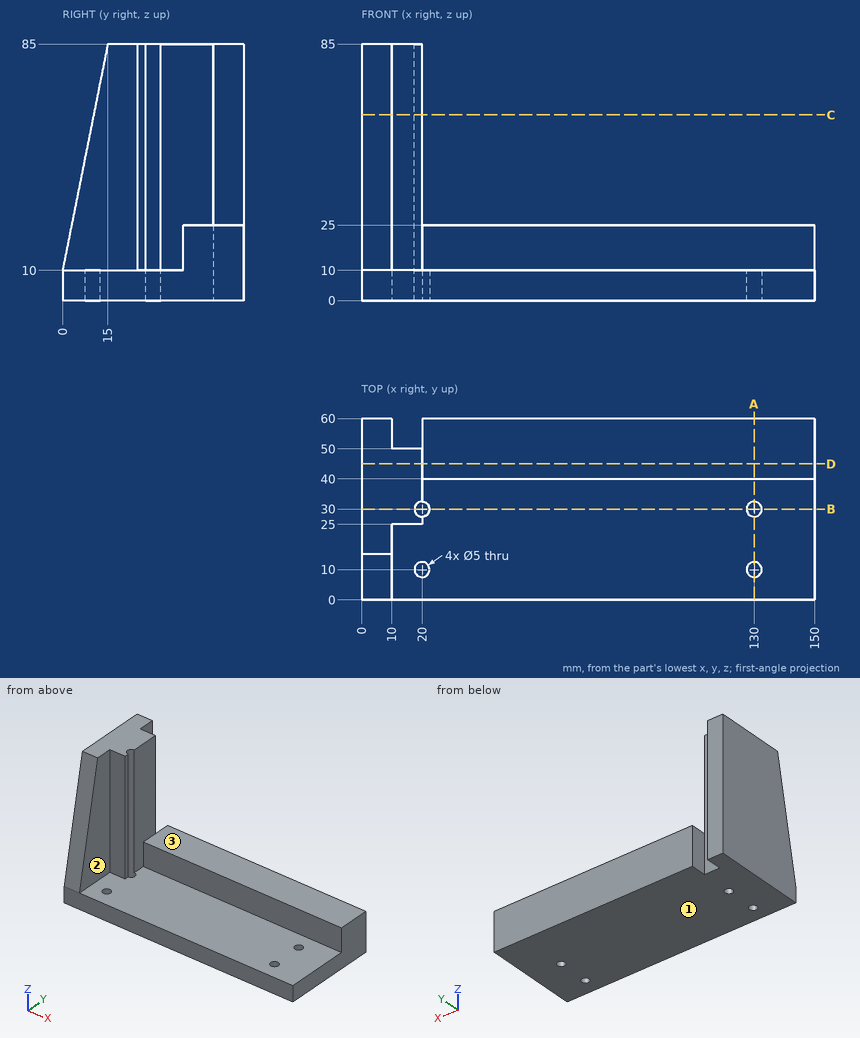
Study the drawing (mm; zero at the part's minimum x, y, z) and answer. A direction names the side the tool comes from. Coordinates: 2 decimals unless noted, no trailing zeros. Write each loop counter-clockwise with the first axis right and the second up, starting at its lowest first coordinate (ties: lowest second). Pieces come first, ordered by that corner, then holes. Notation, with made-up numbers: (-19, 5) - (5, 5) arc R29 cw to (5, 34) - close; hole circle Ø8 at (-30, 8). An arc over 180 degrees is marked (long way). One line per item, written item: value.
1) A tool of negligible diameter and unlimited length cuts with its end or side. For the marked faces 1, 2 and 3, from which of +Z, -Z, +X, -X, +Y, -Y can it reach the whole face along a straight path? Write none if from no direction.
Geometry check:
face 1: -Z, +X, -X, +Y, -Y
face 2: +Z, +X, -Y
face 3: +Z, +X, +Y, -Y
2) Find section D-D (y = 45). Give the vertices of the cut face in (x, z).
Geometry check:
outline: (0, 0) - (150, 0) - (150, 25) - (20, 25) - (20, 85) - (0, 85) - close
3) Find section B-B (y = 30). Give the vertices of the cut face in (x, z), and give its area (3 significant figures).
Geometry check:
outline: (0, 0) - (17.5, 0) - (17.5, 85) - (0, 85) - close; (22.5, 0) - (127.5, 0) - (127.5, 10) - (22.5, 10) - close; (132.5, 0) - (150, 0) - (150, 10) - (132.5, 10) - close
area: 2,710 mm2
4) Each of these flat-tipped pins is pushed along its axis until it touches: pin 1 Ø16.5 at (x, z) = (112, 20) entering from -Y; pin 2 Ø3 at (x, z) = (15, 60) entering from +Y; pin 3 Ø11 at (x, z) = (13, 37.5) entering from -Y. Where does it stop, or does it pass through?
Geometry check:
pin 1: stops at y = 40
pin 2: stops at y = 50
pin 3: stops at y = 4.58
5) Consider line 1 along Y through (x, z) = (130, 3); line 2 along Z through (x, y) = (138.5, 36). Determine where each line is inside the solid, lowest interval first. Write a range as from..to.
Geometry check:
line 1: y = 0..7.5, 12.5..27.5, 32.5..60
line 2: z = 0..10
6) Find section A-A (x = 130). Give the vertices of the cut face in (y, z).
Geometry check:
outline: (0, 0) - (7.5, 0) - (7.5, 10) - (0, 10) - close; (12.5, 0) - (27.5, 0) - (27.5, 10) - (12.5, 10) - close; (32.5, 0) - (60, 0) - (60, 25) - (40, 25) - (40, 10) - (32.5, 10) - close
7) Find section C-C (z = 61.5). Give the vertices of the cut face in (x, y), and give its area (3 significant figures).
Geometry check:
outline: (0, 10.3) - (10, 10.3) - (10, 25) - (20, 25) - (20, 27.5) arc R2.5 cw to (20, 32.5) - (20, 50) - (10, 50) - (10, 60) - (0, 60) - close
area: 737 mm2
